Part model, mm, in its own coordinate system. A direction names the side the tool comes from. Coordinates: 2 decimals unless noted, no trailing zeros. Order: outer loops, then holes, each group sorted by start corner. A loop starts at its lowest first (then second) coordinate and runs counter-clockwise, first axis right, second up.
from build123d import *

# Parameters (mm, degrees)
F0_R     = 10
F1_DEPTH = 40
F2_W     = 48
F2_H     = 38
F2_H_2   = 22
F3_DEPTH = 44.001
F5_DEPTH = 30.001
F6_DEPTH = 10
F7_R     = 8


with BuildPart() as f1:
    # F0 (on Right) → F1 (new body, symmetric)
    with BuildSketch(Plane.YZ):
        with BuildLine():
            Line((-100, 0), (0, 0))
            Line((0, 0), (0, 68))
            ThreePointArc((0, 68), (-22, 90), (-44, 68))
            Line((-44, 68), (-44, 30))
            Line((-44, 30), (-100, 30))
            Line((-100, 30), (-100, 0))
        make_face()
        with Locations((-22, 68)):
            Circle(F0_R, mode=Mode.SUBTRACT)
    extrude(amount=F1_DEPTH, both=True)

    # F2 (on face) → F3 (cut, through all)
    with BuildSketch(Plane.XZ.offset(44)):
        with Locations((0, 49)):
            Rectangle(F2_W, F2_H)
        with Locations((0, 79)):
            Rectangle(F2_W, F2_H_2)
    extrude(amount=-F3_DEPTH, mode=Mode.SUBTRACT)

    # F4 (on face) → F5 (cut, through all)
    with BuildSketch(Plane.XY.offset(30)):
        with BuildLine():
            Line((-8.160617, -76), (-8.160617, -100))
            Line((-8.160617, -100), (8.160617, -100))
            Line((8.160617, -100), (8.160617, -76))
            ThreePointArc((8.160617, -76), (0, -67.839383), (-8.160617, -76))
        make_face()
    extrude(amount=-F5_DEPTH, mode=Mode.SUBTRACT)

    # F4 (on face) → F6 (cut)
    with BuildSketch(Plane.XY.offset(30)):
        with BuildLine():
            Line((-16, -76), (-16, -100))
            Line((-16, -100), (-8.160617, -100))
            Line((-8.160617, -100), (-8.160617, -76))
            ThreePointArc((-8.160617, -76), (0, -67.839383), (8.160617, -76))
            Line((8.160617, -76), (8.160617, -100))
            Line((8.160617, -100), (16, -100))
            Line((16, -100), (16, -76))
            ThreePointArc((16, -76), (0, -60), (-16, -76))
        make_face()
    extrude(amount=-F6_DEPTH, mode=Mode.SUBTRACT)

    # F7
    f7_edges = [f1.edges().sort_by_distance(p)[0] for p in [
        (-40, -100, 15),
        (40, -100, 15),
    ]]
    fillet(f7_edges, radius=F7_R)


solid = f1.part
Q1. Cut at D-D on z = 61. Write the cut outline in (x, y).
Results list:
outline: (-40, -44) - (-24, -44) - (-24, -29.14) - (-40, -29.14) - close; (-40, -14.86) - (-24, -14.86) - (-24, 0) - (-40, 0) - close; (24, -44) - (40, -44) - (40, -29.14) - (24, -29.14) - close; (24, -14.86) - (40, -14.86) - (40, 0) - (24, 0) - close
Q2. Cut at A-A on y = -84.5. Write the cut outline in (x, z), and give its area (3 significant figures).
Results list:
outline: (-40, 0) - (-8.16, 0) - (-8.16, 20) - (-16, 20) - (-16, 30) - (-40, 30) - close; (8.16, 0) - (40, 0) - (40, 30) - (16, 30) - (16, 20) - (8.16, 20) - close
area: 1,750 mm2
Q3. Cut at B-B on z = 45.5. Write the cut outline in (x, y), and give its area (3 significant figures).
Results list:
outline: (-40, -44) - (-24, -44) - (-24, 0) - (-40, 0) - close; (24, -44) - (40, -44) - (40, 0) - (24, 0) - close
area: 1,410 mm2
Q4. Wall check: line 1 along Y through (x, z) = (28.25, 68); line 2 along Z through (x, y) = (30, -22); line 3 along X through (y, z) = (-37, 33). Give the ranges that are in metal, low to high.
Results list:
line 1: y = -44 to -32, -12 to 0
line 2: z = 0 to 58, 78 to 90
line 3: x = -40 to -24, 24 to 40
Q5. Mould opens along Z. For faces 1 (the face through (32, -22, 90)), 2 (the face through (24, -22, 53)), 3 (the face through (31.89, -16.62, 76.43)) say: pulls with the +Z half, pulls with the -Z half, needs draft (parallel to the pull), parting line crosses it, or undercut.
Results list:
face 1: pulls with the +Z half
face 2: needs draft
face 3: undercut
Q6. Pin check, flat tips, straight feed: pin 1 Ø10 at (x, y) = (1, -32.5) entering from -Z; pin 2 Ø13 at (x, z) = (-33, 40.5) entering from -Y; pin 3 Ø9.5 at (x, y) = (-7.5, -84) entering from +Z; pin 4 Ø5 at (x, y) = (-3, -47.5) entering from +Z. Stop position of each tip, or through.
Results list:
pin 1: stops at z = 0
pin 2: stops at y = -44
pin 3: stops at z = 20
pin 4: stops at z = 30
Q7. Which spindle directions (+Z, -Z, +X, -X, +Y, -Y) get a long thin tool onto all of the face, cutting with end or side? Do faces 4 (the face through (-24, -22, 54)), 5 (the face through (32, -44, 49)), 6 (the face through (8.161, -88, 10)), 7 (the face through (16, -88, 25)). Say none if no direction does.
Results list:
face 4: +Z, +Y, -Y
face 5: +Z, +X, -X, -Y
face 6: +Z, -Z, -Y
face 7: +Z, -Y
Q8. Cut at C-C on y = -22. Write the cut outline in (x, z).
Results list:
outline: (-40, 0) - (40, 0) - (40, 58) - (24, 58) - (24, 30) - (-24, 30) - (-24, 58) - (-40, 58) - close; (-40, 78) - (-24, 78) - (-24, 90) - (-40, 90) - close; (24, 78) - (40, 78) - (40, 90) - (24, 90) - close
